Source: CAD feature listing. Evaluate the final solid. Frame: model axes, mm. Round coordinates to 2 decimals unless told otherwise and drop trailing zeros. Loops run counter-clockwise (first coordinate to the right, second up) from the corner with the lowest first, then second, coordinate; pieces in that order, holes last. Notation, with made-up numbers: M 58,-20.75 L 109,-20.75 A23 ccw 109,12.25 Z; hole C 86.25,85 d5. An arc over 180 degrees is marked long. Answer as a JSON object with one key per item and string values.
from build123d import *

# Parameters (mm, degrees)
SKETCH1_W           = 100
SKETCH1_H           = 200
BOSS_EXTRUDE2_DEPTH = 3.18
SKETCH2_R           = 1.55
SKETCH2_W           = 3.18
SKETCH2_H           = 90.125
CUT_EXTRUDE1_DEPTH  = 4.18
SKETCH5_R           = 1.47
CUT_EXTRUDE4_DEPTH  = 4.18
SKETCH6_R           = 1.47
CUT_EXTRUDE5_DEPTH  = 4.18
SKETCH4_W           = 13.35
SKETCH4_H           = 11.35
CUT_EXTRUDE7_DEPTH  = 4.18
SKETCH7_R           = 3.25
CUT_EXTRUDE8_DEPTH  = 4.18


with BuildPart() as part:
    # Sketch1 → Boss-Extrude2 (new body)
    with BuildSketch(Plane.XY):
        Rectangle(SKETCH1_W, SKETCH1_H)
    extrude(amount=BOSS_EXTRUDE2_DEPTH)

    # Sketch2 → Cut-Extrude1 (cut, through all)
    with BuildSketch(Plane.XY.offset(3.18)):
        with Locations((-48, 0)):
            Circle(SKETCH2_R)
        Polygon((-10, 100), (-10, 96.82), (-1.5, 96.82), (-1.5, 92.82), (-3.25, 92.82), (-3.25, 89.82), (-1.5, 89.82), (-1.5, 87), (1.5, 87), (1.5, 89.82), (3.25, 89.82), (3.25, 92.82), (1.5, 92.82), (1.5, 96.82), (10, 96.82), (10, 100), align=None)
        with Locations((-48.41, 54.9375)):
            Rectangle(SKETCH2_W, SKETCH2_H)
        with Locations((-48.41, -54.9375)):
            Rectangle(SKETCH2_W, SKETCH2_H)
    cut_extrude1 = extrude(amount=-CUT_EXTRUDE1_DEPTH, mode=Mode.SUBTRACT)

    # Mirror1: Cut-Extrude1 across plane
    add(cut_extrude1.mirror(Plane.ZX), mode=Mode.SUBTRACT)

    # Mirror3: Cut-Extrude1 across plane
    add(cut_extrude1.mirror(Plane(origin=(0, 0, 0), x_dir=(0, 0, 1), z_dir=(1, 0, 0))), mode=Mode.SUBTRACT)

    # Sketch5 → Cut-Extrude4 (cut, through all)
    with BuildSketch(Plane.XY.offset(3.18)):
        with Locations((-37.58090562, 28.464149283)):
            Circle(SKETCH5_R)
        with Locations((35.904481485, 28.464149283)):
            Circle(SKETCH5_R)
        with Locations((-37.58090562, -26.535850717)):
            Circle(SKETCH5_R)
        with Locations((35.904481485, -26.535850717)):
            Circle(SKETCH5_R)
    extrude(amount=-CUT_EXTRUDE4_DEPTH, mode=Mode.SUBTRACT)

    # Sketch6 → Cut-Extrude5 (cut, through all)
    with BuildSketch(Plane.XY.offset(3.18)):
        with Locations((-5.638260743, 58.12)):
            Circle(SKETCH6_R)
        with Locations((8.111739257, 79.62)):
            Circle(SKETCH6_R)
        with Locations((21.861739257, 58.12)):
            Circle(SKETCH6_R)
    extrude(amount=-CUT_EXTRUDE5_DEPTH, mode=Mode.SUBTRACT)

    # Sketch4 → Cut-Extrude7 (cut, through all)
    with BuildSketch(Plane.XY.offset(3.18)):
        with Locations((-11.677157219, -77.351093612)):
            Rectangle(SKETCH4_W, SKETCH4_H)
    extrude(amount=-CUT_EXTRUDE7_DEPTH, mode=Mode.SUBTRACT)

    # Sketch7 → Cut-Extrude8 (cut, through all)
    with BuildSketch(Plane.XY.offset(3.18)):
        with Locations((-29.760307604, 83.086151576)):
            Circle(SKETCH7_R)
    extrude(amount=-CUT_EXTRUDE8_DEPTH, mode=Mode.SUBTRACT)


solid = part.part
Item 1: Pull-direction query (Y, two-part tool) for faces 1 (the flat face through (-1, 1, 0)), 2 (the cylindrical face through (-30.465, 79.913, 1.612)); classes: pulls with the +Y half, pulls with the -Y half, needs draft (parallel to the pull), parting line crosses it, or undercut.
Answer sheet:
{"face 1": "needs draft", "face 2": "undercut"}
Item 2: Line query: probe 1 along Y at (x, z) = (-3, 2.85); probe 2 along Y at (x, z) = (-11.5, 2.6); probe 3 along Y at (x, z) = (-30, 1.9) (3 decimals). Output: solid intervals per line, ascending. Write a range as from..to.
Answer sheet:
{"probe 1": "y = -96.82..-92.82, -89.82..89.82, 92.82..96.82", "probe 2": "y = -100..-83.03, -71.68..100", "probe 3": "y = -100..79.845, 86.327..100"}
Item 3: Section C-C on y = 35. Return the cut outline in (x, z), then the cut area to 3 significant figures.
Answer sheet:
{"outline": "M -46.82,0 L 46.82,0 L 46.82,3.18 L -46.82,3.18 Z", "area": "298 mm²"}
Item 4: Section A-A on y = -75.5. Return the cut outline in (x, z), then the cut area to 3 significant figures.
Answer sheet:
{"outline": "M -46.82,0 L -18.35,0 L -18.35,3.18 L -46.82,3.18 Z; M -5,0 L 46.82,0 L 46.82,3.18 L -5,3.18 Z", "area": "255 mm²"}
Item 5: Section B-B on x = -29.5. Return the cut outline in (y, z), then the cut area to 3 significant figures.
Answer sheet:
{"outline": "M -100,0 L 79.85,0 L 79.85,3.18 L -100,3.18 Z; M 86.33,0 L 100,0 L 100,3.18 L 86.33,3.18 Z", "area": "615 mm²"}
Item 6: Section D-D on z = 2.45. Give the number of separate pieces and of enclosed holes in the cut face, then the cut area to 3 significant figures.
Answer sheet:
{"separate pieces": "1", "enclosed holes": "11", "area": "18,400 mm²"}
Item 7: Contact query for flat-ended pins moving along their axis: pin 1 Ø1 at (x, z) = (-48, 1) entering from -Y (3 decimals); pin 2 Ø0.9 at (x, z) = (-2.5, 2) entering from +Y; pin 3 Ø0.8 at (y, z) = (88.5, 1.5) entering from -X. Output: stop coordinate, or through.
Answer sheet:
{"pin 1": "stops at y = -9.875", "pin 2": "stops at y = 96.82", "pin 3": "stops at x = -46.82"}
